Check sheet for the modelled part. Datum: model origin and axes. Units: mm. Give positions to 0.01 mm unless a question says otherwise; leave off trailing zeros. Order: outer loops, then holes, each group sorted by start corner. A loop starts at its lowest first (then second) coordinate and runs counter-clockwise, first axis right, second up.
```python
from build123d import *

# Parameters (mm, degrees)
SKETCH005_R      = 2.1
EXTRUDE004_DEPTH = 10
BOX011_W         = 8
BOX011_H         = 60
BOX011_DEPTH     = 13
FILLET007_R      = 4


with BuildPart() as obj1:
    # Sketch005 (on Face2 of Box011) → Extrude004 (new body)
    with BuildSketch(Plane(origin=(18.2, 17.6, -2.4), x_dir=(0, -1, 0), z_dir=(-1, 0, 0))):
        with Locations((3.8, 3.8)):
            Circle(SKETCH005_R)
        with Locations((39.8, 3.8)):
            Circle(SKETCH005_R)
    extrude(amount=EXTRUDE004_DEPTH)


with BuildPart() as obj2:
    # Box011 → Box011 (new body)
    with BuildSketch(Plane(origin=(10.2, -35, -3), x_dir=(1, 0, 0), z_dir=(0, 0, 1))):
        with Locations((4, 30)):
            Rectangle(BOX011_W, BOX011_H)
    extrude(amount=BOX011_DEPTH)

    # Fillet007
    fillet007_edges = [obj2.edges().sort_by_distance(p)[0] for p in [
        (14.2, -35, -3),
        (14.2, 25, -3),
    ]]
    fillet(fillet007_edges, radius=FILLET007_R)

    # Cut006: cut obj1
    add(obj1.part, mode=Mode.SUBTRACT)


solid = obj2.part
```
(1) Sectioned sample at A-A (y = -22.2). Enter the section's corners in (x, z), plus the area to 3 significant figures.
(2) Sectioned sample at C-C (z = 2.5). Enter the section's corners in (x, y), plus the area to 3 significant figures.
(3) Thickness scan on L1, parallel to Y at x = 15, z = 1.4; L2, parallel to Z at x = 15, y = 13.8; L3, parallel to Y at x = 12.75, z = -1. Record the ranges inside material, lowest first.
(4) Go/stop test with flat-tipped pins: P1, Ø5, axis at y = -22.2, z = 1.4, coming from the -X side; P2, Ø3.5, axis at y = 13.8, z = 1.4, coming from the +X side. Record where each tip stops, or that it passes through.
(5) Release check for a two-part mould opening along Z. For faces 1 (the face through (14.256, -33.859, -1.797)), 2 (the face through (14, -35, 5)), 3 (the face through (14.26, -20.1, 1.49)) record: released by +Z, released by -Z, zero draft, split by the parting line, or undercut.
(6) Sectioned sample at B-B (x = 13.75). Enter the section's corners in (y, z).
(7) Sectioned sample at D-D (z = -2). Enter the section's corners in (x, y), plus the area to 3 significant figures.
Values follow:
1. outline: (10.2, -3) - (18.2, -3) - (18.2, -0.7) - (10.2, -0.7) - close; (10.2, 3.5) - (18.2, 3.5) - (18.2, 10) - (10.2, 10) - close
1. area: 70.4 mm2
2. outline: (10.2, -35) - (18.2, -35) - (18.2, -23.99) - (10.2, -23.99) - close; (10.2, -20.41) - (18.2, -20.41) - (18.2, 12.01) - (10.2, 12.01) - close; (10.2, 15.59) - (18.2, 15.59) - (18.2, 25) - (10.2, 25) - close
2. area: 423 mm2
3. L1: y = -35 to -24.3, -20.1 to 11.7, 15.9 to 25
3. L2: z = -3 to -0.7, 3.5 to 10
3. L3: y = -34.46 to 24.46
4. P1: stops at x = 10.2
4. P2: passes through
5. face 1: released by -Z
5. face 2: zero draft
5. face 3: undercut
6. outline: (-35, 1) arc R4 ccw to (-31, -3) - (21, -3) arc R4 ccw to (25, 1) - (25, 10) - (-35, 10) - close; hole circle Ø4.2 at (-22.2, 1.4); hole circle Ø4.2 at (13.8, 1.4)
7. outline: (10.2, -33.65) - (18.2, -33.65) - (18.2, 23.65) - (10.2, 23.65) - close
7. area: 458 mm2
